Work out the finished part from the listing and answer in its coordinate system (mm). A direction names the side the tool comes from. Give positions to 0.01 mm unless a question says otherwise; leave off trailing zeros. Loops run counter-clockwise (first coordinate to the right, second up) from the corner with the lowest first, then second, coordinate; pieces in that order, holes last. Notation, with made-up numbers: M 17,72 L 32,72 A16 ccw 32,88 Z; hole C 75.5,10.25 d8. An arc over 180 degrees is marked long. Write item = value, one per line. Start each with the question number.
1. Section B-B on z = -346.5 is taken. Determine the outline of the cut face in (x, y).
2. The mould has two halves that part along X. Classify faces 1 (the face through (145.87, 5.44, 526.92)), 2 (the face through (-257.03, 4.93, 536.14)), 3 (the face through (153.372, 4.93, 534.264)): released by +X, released by -X, zero draft, split by the parting line, or undercut.
3. Section D-D on z = 460 is taken. Determine the outline of the cut face in (x, y).
4. Consider L1, parallel to X at y = 3.25, z = 385; L2, parallel to X at y = 8.75, z = 64; L3, parallel to Z at x = -138, y = 1.25. Determine where each line is inside the solid, lowest interval first. Write a range as [from, to].
5. Section A-A on y = 5.75 is taken. Determine the outline of the cut face in (x, z), plus the area to 3 significant figures.
6. Section C-C on x = -42.5 is taken. Determine the outline of the cut face in (y, z), plus the area to 3 significant figures.
7. For faces 4 (the face through (-285, 0, 176)), 5 (the face through (151.15, 5.44, 535.78)), 6 (the face through (143.81, 4.93, 528.27)), determine the directions among +Z, -Z, +X, -X, +Y, -Y from which every point of the face is accessible in a straight line to the end or side of a thin tool.
8. Flat-ended cylindrical pins translate along their axes: pin 1 Ø2.5 at (y, z) = (4, -160) entering from +X; pin 2 Ø6 at (x, y) = (1, 4) entering from -Z. Find the tip coordinate at first contact, or state that the pin passes through.
```python
from build123d import *

# Parameters (mm, degrees)
F1_DEPTH = 10
F2_DEPTH = 1
F3_DEPTH = 700


with BuildPart() as f1:
    # F0 (on Front) → F1 (new body)
    with BuildSketch(Plane.XZ):
        with BuildLine():
            Line((67.234268, 570.5), (-172.765732, 570.5))
            ThreePointArc((-172.765732, 570.5), (-257.972099, 535.206367), (-293.265732, 450))
            Line((-293.265732, 450), (-293.265732, -450))
            Line((-293.265732, -450), (-292.765732, -450))
            Line((-292.765732, -450), (-292.765732, 450))
            ThreePointArc((-292.765732, 450), (-257.618545, 534.852814), (-172.765732, 570))
            Line((-172.765732, 570), (67.234268, 570))
            ThreePointArc((67.234268, 570), (152.087082, 534.852814), (187.234268, 450))
            Line((187.234268, 450), (187.234268, -450))
            Line((187.234268, -450), (187.734268, -450))
            Line((187.734268, -450), (187.734268, 450))
            ThreePointArc((187.734268, 450), (152.440635, 535.206367), (67.234268, 570.5))
        make_face()
        with BuildLine():
            Line((-282.765732, 450), (-282.765732, -450))
            Line((-282.765732, -450), (-282.265732, -450))
            Line((-282.265732, -450), (-282.265732, 450))
            ThreePointArc((-282.265732, 450), (-250.193924, 527.428193), (-172.765732, 559.5))
            Line((-172.765732, 559.5), (67.234268, 559.5))
            ThreePointArc((67.234268, 559.5), (144.662461, 527.428193), (176.734268, 450))
            Line((176.734268, 450), (176.734268, -450))
            Line((176.734268, -450), (177.234268, -450))
            Line((177.234268, -450), (177.234268, 450))
            ThreePointArc((177.234268, 450), (145.016014, 527.781746), (67.234268, 560))
            Line((67.234268, 560), (-172.765732, 560))
            ThreePointArc((-172.765732, 560), (-250.547478, 527.781746), (-282.765732, 450))
        make_face()
    extrude(amount=-F1_DEPTH)

    # F0 (on Front) → F2 (join)
    with BuildSketch(Plane.XZ):
        with BuildLine():
            Line((-292.765732, 450), (-292.765732, -450))
            Line((-292.765732, -450), (-282.765732, -450))
            Line((-282.765732, -450), (-282.765732, 450))
            ThreePointArc((-282.765732, 450), (-250.547478, 527.781746), (-172.765732, 560))
            Line((-172.765732, 560), (67.234268, 560))
            ThreePointArc((67.234268, 560), (145.016014, 527.781746), (177.234268, 450))
            Line((177.234268, 450), (177.234268, -450))
            Line((177.234268, -450), (187.234268, -450))
            Line((187.234268, -450), (187.234268, 450))
            ThreePointArc((187.234268, 450), (152.087082, 534.852814), (67.234268, 570))
            Line((67.234268, 570), (-172.765732, 570))
            ThreePointArc((-172.765732, 570), (-257.618545, 534.852814), (-292.765732, 450))
        make_face()
    extrude(amount=-F2_DEPTH)

    # F2_face (on face) → F3 (cut)
    with BuildSketch(Plane(origin=(182.234268, 2.75, -450), x_dir=(1, 0, 0), z_dir=(0, 0, -1))):
        Polygon((5, 1.75), (5, -7.25), (5.5, -7.25), (5.5, 2.75), (-5.5, 2.75), (-5.5, -7.25), (-5, -7.25), (-5, 1.75), align=None)
    extrude(amount=-F3_DEPTH, mode=Mode.SUBTRACT)


solid = f1.part
```
Verdict:
q1.outline = M -293.27,0 L -282.27,0 L -282.27,10 L -282.77,10 L -282.77,1 L -292.77,1 L -292.77,10 L -293.27,10 Z
q2.face_1 = undercut
q2.face_2 = released by -X
q2.face_3 = released by +X
q3.outline = M -292.85,0 L -281.81,0 L -281.81,10 L -282.31,10 L -282.31,1 L -292.35,1 L -292.35,10 L -292.85,10 Z; M 176.28,0 L 187.32,0 L 187.32,10 L 186.82,10 L 186.82,1 L 176.78,1 L 176.78,10 L 176.28,10 Z
q4.L1 = [-293.27, -292.77], [-282.77, -282.27], [176.73, 177.23], [187.23, 187.73]
q4.L2 = [-293.27, -292.77], [-282.77, -282.27]
q4.L3 = [559.5, 560], [570, 570.5]
q5.outline = M -293.27,-450 L -292.77,-450 L -292.77,450 A120 cw -172.77,570 L 67.23,570 A120 cw 187.23,450 L 187.23,250 L 187.73,250 L 187.73,450 A120.5 ccw 67.23,570.5 L -172.77,570.5 A120.5 ccw -293.27,450 Z; M -282.77,-450 L -282.27,-450 L -282.27,450 A109.5 cw -172.77,559.5 L 67.23,559.5 A109.5 cw 176.73,450 L 176.73,250 L 177.23,250 L 177.23,450 A110 ccw 67.23,560 L -172.77,560 A110 ccw -282.77,450 Z
q5.area = 1,700 mm2
q6.outline = M 0,559.5 L 10,559.5 L 10,560 L 1,560 L 1,570 L 10,570 L 10,570.5 L 0,570.5 Z
q6.area = 20.0 mm2
q7.face_4 = +Z, -Z, +X, -X, -Y
q7.face_5 = +Y
q7.face_6 = -Z, +Y, -Y
q8.pin_1 = -282.27
q8.pin_2 = 559.5
